Model file for the job. Use its own axes, mm. Face numbers are marked on the shaded views. Coordinates: 2 decimals unless noted, no trailing zeros. Loops run counter-clockwise (first coordinate to the right, second up) from the corner with the lowest first, then second, coordinate; pieces in that order, holes last. Notation, with made-up numbers: (-20, -34.75) -> (19, -34.75) arc R34 cw to (19, 3.25) -> close; hole circle Ø2 at (-2.75, 74.5). An arc over 180 degrees is marked (long way). Use one line per item in the form item = value.
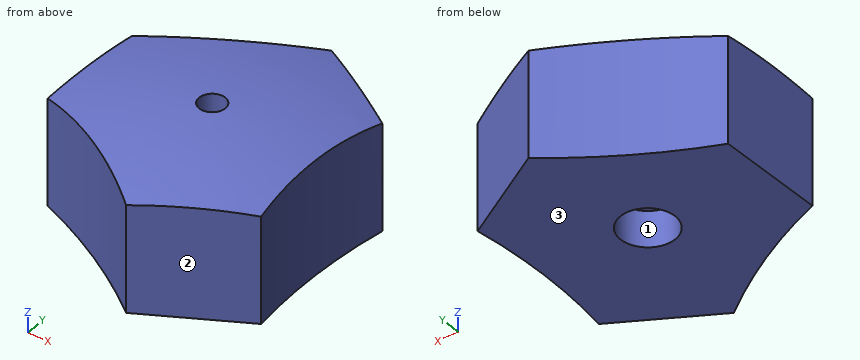
```python
from build123d import *

# Parameters (mm, degrees)
BOSS_EXTRUDE1_DEPTH = 13.75
SKETCH4_R           = 3.05
CUT_EXTRUDE1_DEPTH  = 4
SKETCH5_R           = 1.45
CUT_EXTRUDE2_DEPTH  = 139.272786048


with BuildPart() as part:
    # Boss-Extrude1: read off the stored shape, not the designer's step
    # Boss-Extrude1 outline → Boss-Extrude1 (new body)
    with BuildSketch(Plane.XY):
        with BuildLine():
            Line((-44.963090762, -123.889928328), (-34.25904674, -117.947860363))
            ThreePointArc((-34.25904674, -117.947860363), (-34.937745159, -108.915491102), (-34.292771341, -99.880651048))
            Line((-34.292771341, -99.880651048), (-44.790775161, -93.581710984))
            ThreePointArc((-44.790775161, -93.581710984), (-52.273687189, -98.685665687), (-60.420575103, -102.644522003))
            Line((-60.420575103, -102.644522003), (-60.626615305, -114.885530032))
            ThreePointArc((-60.626615305, -114.885530032), (-52.465004859, -118.81394459), (-44.963090762, -123.889928328))
        make_face()
    extrude(amount=BOSS_EXTRUDE1_DEPTH)

    # Boss-Extrude1 2 outline → Boss-Extrude1 2 (revolve, cut)
    with BuildSketch(Plane(origin=(-46.558812402, -108.805033793, 0), x_dir=(1, 0, 0), z_dir=(0, -1, 0))):
        with BuildLine():
            ThreePointArc((0, 13.75), (7.723984527, 13.263031911), (15.32564925, 11.809839448))
            Line((15.32564925, 11.809839448), (15.32564925, 13.75))
            Line((15.32564925, 13.75), (0, 13.75))
        make_face()
    revolve(axis=Axis((-46.558812402, -108.805033793, 0), (0, 0, 1)), mode=Mode.SUBTRACT)

    # Sketch4 → Cut-Extrude1 (cut)
    with BuildSketch(Plane(origin=(0, 0, 0), x_dir=(-1, 0, 0), z_dir=(0, 0, -1))):
        with Locations((46.784528167, -108.691568131)):
            Circle(SKETCH4_R)
    extrude(amount=-CUT_EXTRUDE1_DEPTH, mode=Mode.SUBTRACT)

    # Sketch5 → Cut-Extrude2 (cut, through all)
    with BuildSketch(Plane(origin=(0, 0, 4), x_dir=(-1, 0, 0), z_dir=(0, 0, -1))):
        with Locations((46.784528167, -108.691568131)):
            Circle(SKETCH5_R)
    extrude(amount=-CUT_EXTRUDE2_DEPTH, mode=Mode.SUBTRACT)


solid = part.part
```
Q1. Mould opens along X. For the marked faces 1, 2 and 3 say: released by +X, released by -X, zero draft, split by the parting line, or undercut.
Result:
face_1 = undercut
face_2 = released by +X
face_3 = zero draft
Q2. Wall check: line 1 along X through (y, z) = (-108.5, 8); line 2 along X through (y, z) = (-120, 11.5); line 3 along Y through (x, z) = (-59, 7.25). Give the ranges that are in metal, low to high.
Result:
line_1 = -60.52 to -48.22, -45.35 to -34.94
line_2 = -50.49 to -37.96
line_3 = -115.55 to -102.06
Q3. Band-saw the part on B-B, the plane z = 4.5. Write the cut outline in (x, y), and give its area (3 significant figures).
Result:
outline = (-60.63, -114.89) arc R61.98 cw to (-44.96, -123.89) -> (-34.26, -117.95) arc R61.98 cw to (-34.29, -99.88) -> (-44.79, -93.58) arc R61.98 cw to (-60.42, -102.64) -> close; hole circle Ø2.9 at (-46.78, -108.69)
area = 559 mm2
Q4. Band-saw the part on A-A, the plane y = -108. Write the cut outline in (x, z), and give its area (3 significant figures).
Result:
outline = (-60.51, 0) -> (-49.76, 0) -> (-49.76, 4) -> (-48.06, 4) -> (-48.06, 13.73) arc R61.49 ccw to (-60.51, 12.14) -> close; (-45.51, 4) -> (-43.81, 4) -> (-43.81, 0) -> (-34.93, 0) -> (-34.93, 12.64) arc R61.49 ccw to (-45.51, 13.74) -> close
area = 291 mm2
Q5. Pin check, flat tips, straight feed: pin 1 Ø6 at (x, y) = (-39.5, -97.5) entering from -Z; pin 2 Ø5 at (x, z) = (-42.5, 7.5) entering from -Y; pin 3 Ø5 at (x, z) = (-49.5, 3) entering from -Y; pin 4 Ø1.5 at (y, z) = (-103, 4.5) entering from +X. Stop position of each tip, or through.
Result:
pin_1 = 0
pin_2 = -123.89
pin_3 = -122.35
pin_4 = -34.59
Q6. Band-saw the part on C-C, the plane x = -57.75. Write the cut outline in (y, z), and give its area (3 significant figures).
Result:
outline = (-116.1, 0) -> (-101.51, 0) -> (-101.51, 12.28) arc R60.47 ccw to (-116.1, 12.28) -> close
area = 184 mm2
Q7. Band-saw the part on D-D, the plane z = 1. Write the cut outline in (x, y).
Result:
outline = (-60.63, -114.89) arc R61.98 cw to (-44.96, -123.89) -> (-34.26, -117.95) arc R61.98 cw to (-34.29, -99.88) -> (-44.79, -93.58) arc R61.98 cw to (-60.42, -102.64) -> close; hole circle Ø6.1 at (-46.78, -108.69)
